Part print with two shaded views. Sizes in mm from the minimum x, y, z corner. Coordinates: 2 decimals unless noted, no trailing zeros. Write each loop counter-clockwise with the first axis right and the second up, starting at its lowest first coordinate (ties: lowest second). Pieces come first, ordered by that corner, then holes. Notation, with made-up numbers: M 36,4.25 L 87,4.25 A19 ccw 87,27.25 Z; hole C 73.5,-5.75 d11. An arc over 180 degrees is marked long. One line per question, with ' | ' between items. Start each with the question number.
(1) Cut at D-D (x = 37). Write the cut outline in (y, z).
(2) Flat gauge pins, fed straight in: pin 1 Ø5 at (x, z) = (92.5, 10.5) entering from +Y; pin 2 Ø10 at (x, y) = (55, 14.5) entering from -Z; pin 3 Ø4 at (x, y) = (59, 8) entering from +Z. Where does each tip first touch, or does it go through?
(3) Cut at A-A (y = 9). Write the cut outline in (x, z).
(4) Cut at B-B (z = 21.25). Write the cut outline in (x, y), plus the area to 3 significant figures.
(5) Wall check: probe 1 along X at (y, z) = (13.25, 23.5); probe 2 along Z at (x, y) = (60, 8.75); probe 3 along Y at (x, z) = (69.5, 3.75). Give the ranges that are in metal, low to high.
(6) Cut at C-C (x = 50). Write the cut outline in (y, z), plus the area to 3 significant figures.
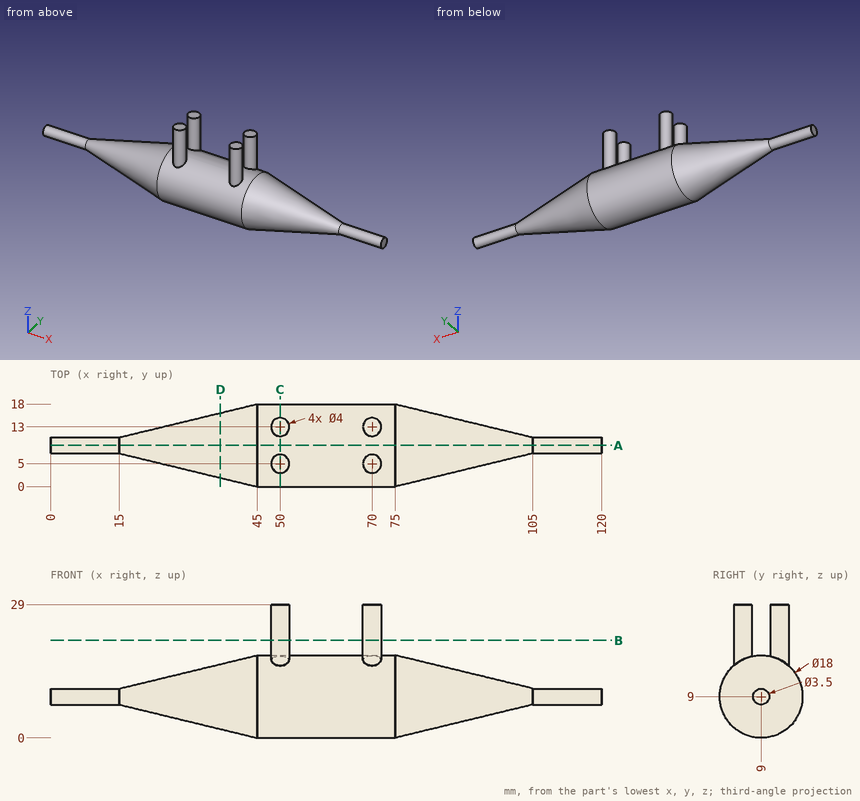
Filled in:
1) outline: C 9,9 d14.13
2) pin 1: y = 14.3 | pin 2: z = 0.01 | pin 3: z = 18
3) outline: M 0,7.25 L 15,7.25 L 45,0 L 75,0 L 105,7.25 L 120,7.25 L 120,10.75 L 105,10.75 L 75,18 L 45,18 L 15,10.75 L 0,10.75 Z
4) outline: C 50,5 d4; C 50,13 d4; C 70,5 d4; C 70,13 d4 | area: 50.3 mm²
5) probe 1: 48.02 to 51.98, 68.02 to 71.98 | probe 2: 0 to 18 | probe 3: 1.69 to 16.31
6) outline: M 3,15.71 A9 ccw long 15,15.71 L 15,29 L 11,29 L 11,17.77 A9 ccw 7,17.77 L 7,29 L 3,29 Z | area: 351 mm²
